CAD build for the part. Positions are in the model's coordinates, mm. Face numbers are marked on the shaded views. A direction names the side the tool comes from. Give positions to 0.01 mm unless a question says otherwise; leave off trailing zeros. Write each loop counter-clockwise with the first axis right and the second up, starting at its lowest first coordinate (ties: lowest second). Pieces come first, ordered by that corner, then holes. Notation, with made-up numbers: (-32.5, -16) -> (4.5, -16) arc R25 cw to (4.5, 6) -> close; hole circle Ø1 at (53, -30). An arc over 180 degrees is marked (long way). Answer as a JSON object with one key per item and string values.
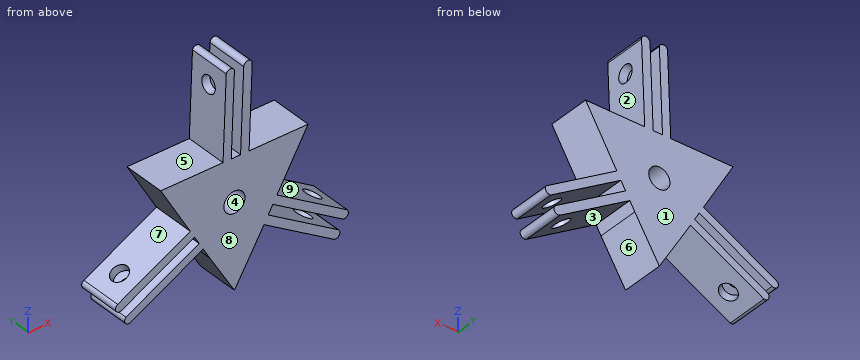
```python
from build123d import *

# Parameters (mm, degrees)
SKETCH1_R           = 2.5
BOSS_EXTRUDE1_DEPTH = 10
SKETCH2_R           = 2
CUT_EXTRUDE1_DEPTH  = 10
CIRPATTERN1_COUNT   = 3
SKETCH3_R           = 2.5
BOSS_EXTRUDE3_DEPTH = 10
SKETCH4_R           = 2.500796224
BOSS_EXTRUDE4_DEPTH = 10


with BuildPart() as part:
    # Sketch1 → Boss-Extrude1 (new body)
    with BuildSketch(Plane(origin=(0, 0, 0), x_dir=(1, 0, 0), z_dir=(0, 1, 0))):
        with BuildLine():
            Line((3.42943918, -9.393558799), (4.197898245, -29.378790113))
            ThreePointArc((4.197898245, -29.378790113), (3.237059632, -30.416474632), (2.199375114, -29.455636019))
            Line((2.199375114, -29.455636019), (1.447231615, -9.894721858))
            ThreePointArc((1.447231615, -9.894721858), (0.350023332, -9.993872306), (-0.751433173, -9.971727442))
            Line((-0.751433173, -9.971727442), (0.000999669, -29.540166516))
            ThreePointArc((0.000999669, -29.540166516), (-0.935779597, -30.318112399), (-1.929530696, -29.614398009))
            Line((-1.929530696, -29.614398009), (-2.697989761, -9.629166695))
            ThreePointArc((-2.697989761, -9.629166695), (-8.461744243, -5.329060364), (-9.849780142, 1.726797949))
            Line((-9.849780142, 1.726797949), (-27.541727692, 11.053908534))
            ThreePointArc((-27.541727692, 11.053908534), (-27.959969541, 12.404861441), (-26.609016634, 12.823103289))
            Line((-26.609016634, 12.823103289), (-9.2926963, 3.694021585))
            ThreePointArc((-9.2926963, 3.694021585), (-8.829958965, 4.693807055), (-8.260052699, 5.636623938))
            Line((-8.260052699, 5.636623938), (-25.58303447, 14.769217519))
            ThreePointArc((-25.58303447, 14.769217519), (-25.788365734, 15.969465103), (-24.682055646, 16.478221605))
            Line((-24.682055646, 16.478221605), (-6.990108095, 7.15111102))
            ThreePointArc((-6.990108095, 7.15111102), (-0.384229532, 9.992615657), (6.420340962, 7.66676085))
            Line((6.420340962, 7.66676085), (23.343829448, 18.324881579))
            ThreePointArc((23.343829448, 18.324881579), (24.722909908, 18.011613191), (24.40964152, 16.63253273))
            Line((24.40964152, 16.63253273), (7.845464685, 6.200700273))
            ThreePointArc((7.845464685, 6.200700273), (8.479935633, 5.300065251), (9.011485871, 4.335103505))
            Line((9.011485871, 4.335103505), (25.582034801, 14.770948997))
            ThreePointArc((25.582034801, 14.770948997), (26.724145331, 14.348647296), (26.611586342, 13.136176404))
            Line((26.611586342, 13.136176404), (9.688097856, 2.478055676))
            ThreePointArc((9.688097856, 2.478055676), (8.845973775, -4.663555293), (3.42943918, -9.393558799))
        make_face()
        Circle(SKETCH1_R, mode=Mode.SUBTRACT)
    extrude(amount=BOSS_EXTRUDE1_DEPTH)

    # Sketch2 → Cut-Extrude1 (cut)
    with BuildSketch(Plane(origin=(3.063714471, 0, -0.117803948), x_dir=(-0.038422953, 0, -0.999261566), z_dir=(0.999261566, 0, -0.038422953))):
        with Locations((-24.518391454, 5)):
            Circle(SKETCH2_R)
    cut_extrude1 = extrude(amount=-CUT_EXTRUDE1_DEPTH, mode=Mode.SUBTRACT)

    # CirPattern1: Cut-Extrude1 ×3 about axis
    cirpattern1_axis = Axis((0, 10, 0), (0, -1, 0))
    for i in range(1, CIRPATTERN1_COUNT):
        add(cut_extrude1.rotate(cirpattern1_axis, i * 360 / CIRPATTERN1_COUNT), mode=Mode.SUBTRACT)

    # Sketch3 → Boss-Extrude3 (add)
    with BuildSketch(Plane(origin=(0, 10, 0), x_dir=(1, 0, 0), z_dir=(0, 1, 0))):
        Polygon((11.5901527, 0), (5.79507635, 10.037366672), (-5.79507635, 10.037366672), (-11.5901527, 0), (-5.79507635, -10.037366672), (5.79507635, -10.037366672), align=None)
        Circle(SKETCH3_R, mode=Mode.SUBTRACT)
    extrude(amount=-BOSS_EXTRUDE3_DEPTH)

    # Sketch4 → Boss-Extrude4 (add)
    with BuildSketch(Plane(origin=(0, 10, 0), x_dir=(1, 0, 0), z_dir=(0, 1, 0))):
        Polygon((-5.79507635, 10.037366672), (0, 19.724396452), (5.79507635, 10.037366672), (11.5901527, 0), (17.38522905, -10.037366672), (5.79507635, -10.037366672), (-5.79507635, -10.037366672), (-17.38522905, -10.037366672), (-11.5901527, 0), align=None)
        Circle(SKETCH4_R, mode=Mode.SUBTRACT)
    extrude(amount=-BOSS_EXTRUDE4_DEPTH)


solid = part.part
```
1) 3-axis set-ups, long thin cutter, end or side, ignore diameter. For the marked faces 5, 6, 7, 8 and 9: which of +Z, -Z, +X, -X, +Y, -Y reach the whole face in a straight line?
Model answer:
{"face 5": "+Z, -X, +Y, -Y", "face 6": "-Z, +Y, -Y", "face 7": "-X, +Y, -Y", "face 8": "+Z, -Z, +X, -X, -Y", "face 9": "+X, +Y, -Y"}
2) Wall check: probe 1 along Z at (x, y) = (-14, 9.25); probe 2 along X at (y, z) = (6, 0); probe 3 along X at (y, z) = (2.25, -11.5). Give the ranges that are in metal, low to high.
Model answer:
{"probe 1": "z = -10.85 to -8.66, -6.18 to -3.91, 4.17 to 10.04", "probe 2": "x = -11.59 to -2.5, 2.5 to 11.59", "probe 3": "x = -27.97 to -24.1, -19.38 to -15.24, -4.92 to 4.92, 12.51 to 16.26, 20.39 to 24.01"}
3) Slice it at C-C (z = 0). List the corners of the cut face in (x, y), then the cut area to 3 significant figures.
Model answer:
{"outline": "(-11.59, 0) -> (-2.5, 0) -> (-2.5, 10) -> (-11.59, 10) -> close; (2.5, 0) -> (11.59, 0) -> (11.59, 10) -> (2.5, 10) -> close", "area": "182 mm2"}
4) Pin check, flat tips, straight feed: pin 1 (2 mm diameter, centred on y = 4, z = 14, fed in from -X); pin 2 (5 mm diameter, centred on y = 3, z = -7.5, fed in from +X); pin 3 (2.5 mm diameter, centred on x = 0.5, y = 5, fed in from +Z). Stop position of each tip, or through.
Model answer:
{"pin 1": "stops at x = -2.57", "pin 2": "stops at x = 21.63", "pin 3": "stops at z = 30.29"}
5) Mould opens along X. For the marked faces 1, 2, 3 and 4 say: released by +X, released by -X, zero draft, split by the parting line, or undercut.
Model answer:
{"face 1": "zero draft", "face 2": "released by +X", "face 3": "undercut", "face 4": "undercut"}
6) Slice it at D-D (x = -3.5). List the corners of the cut face in (y, z), then the cut area to 3 significant figures.
Model answer:
{"outline": "(0, -13.87) -> (10, -13.87) -> (10, 10.04) -> (0, 10.04) -> close", "area": "239 mm2"}
7) Slice it at B-B (z = 27.5). List the corners of the cut face in (x, y), then the cut area to 3 significant figures.
Model answer:
{"outline": "(-2.01, 0) -> (-0.08, 0) -> (-0.08, 10) -> (-2.01, 10) -> close; (2.12, 0) -> (4.13, 0) -> (4.13, 10) -> (2.12, 10) -> close", "area": "39.3 mm2"}
